Autodesk Inventor part; units mm, degrees
ref_plane "YZ Plane" through (0, 0, 0) normal (1, 0, 0) x (0, 1, 0)
ref_plane "XZ Plane" through (0, 0, 0) normal (0, 1, 0) x (-1, 0, 0)
ref_plane "XY Plane" through (0, 0, 0) normal (0, 0, 1) x (1, 0, 0)
sketch "Sketch1" plane through (0, 0, 0) normal (0, 1, 0) x (-1, 0, 0)
  arc A0 (0, 5) -> (0, -5) centre (0, 0) ccw
  arc A1 (-1.6, 1.2) -> (1.6, 1.2) centre (0, 0) ccw
  line L0 (-1.6, 1.2) -> (1.6, 1.2)
  line L1 (95, 124.2688) -> (95, -104.3981) construction
  circle A2 centre (190, 0) radius 11
  arc A3 (179.0531, -6.0345) -> (179.7419, 7.1429) centre (190, 0) ccw
  line L2 (0, -5) -> (177.3016, -5)
  line L3 (0, 5) -> (175.6386, 5)
  arc A4 (179.0531, -6.0345) -> (177.3016, -5) centre (177.3016, -7) ccw
  arc A5 (175.6386, 5) -> (179.7419, 7.1429) centre (175.6386, 10) ccw
  point P0 (178.5436, -5)
  point P1 (178.5436, 5)
  dimension "d2" = 10
  dimension "d3" = 4
  dimension "d4" = 1.2
  dimension "d5" = 95
  dimension "d8" = 22
  dimension "d9" = 25
  dimension "d20" = 2
  dimension "d21" = 5
extrude "Extrusion2" add sketch "Sketch1" along normal blind 10
sketch "Sketch2" plane through (0, 10, 0) normal (0, 1, 0) x (1, 0, 0)
  circle A0 centre (0, 0) radius 2.35
  dimension "d12" = 4.7
extrude "Extrusion3" add sketch "Sketch2" along normal blind 7
sketch "Sketch3" plane through (0, 10, 0) normal (0, 1, 0) x (1, 0, 0)
  circle A0 centre (-190, 0) radius 11 construction
  line L0 (-179, 0) -> (-201, 0) construction
  circle A1 centre (-190, 0) radius 11
  circle A2 centre (-190, 0) radius 3
  point P0 (0, 0)
  dimension "d15" = 22
  dimension "d16" = 22
  dimension "d17" = 6
extrude "Extrusion4" add sketch "Sketch3" against normal blind 3
equation "\"d16\" = d15"
properties part number "eslabon1" material "Plástico ABS"
Can you work these out from the model? Positions are in its coordinate system, mm. A direction names the side the tool comes from. Round coordinates to 2 decimals unless told otherwise and drop trailing zeros. Loops run counter-clockwise (first coordinate to the right, second up) from the corner with the lowest first, then second, coordinate; pieces in that order, holes last. Notation, with made-up numbers: M 9,-39 L 41,-39 A14 ccw 41,-19 Z; hole C -31,81 d5. An arc over 180 degrees is marked long. Write item = value, one per line. Start each with the question number.
(1) Which directions (+Z, -Z, +X, -X, +Y, -Y) give clear straight access to the entire face, cutting with the end or side of a thin tool? Please do faces 5 (the face through (-87, 5, 5)), 6 (the face through (-0.509, 13.451, -2.294)), 7 (the face through (5, 5, 0)), 8 (the face through (-179, 3, 0)), 9 (the face through (-91, 0, 0)).
(2) Suppose I cut it at A-A on x = -190. Write out the boundary of the cut face in (y, z), plus the area to 3 significant figures.
(3) I'm going to push flat-ended pins straight in: P1, Ø4, axis at x = -67.5, y = 7, coming from the +Z side; P2, Ø8, axis at x = -24.5, y = 5.5, coming from the -Z side; P3, Ø7.5, axis at x = -70.5, z = 1.5, coming from the +Y side. Where does each tip first touch, or does it pass through?
(4) I need wall thicknesses on line 1 along X through (y, z) = (4.75, 0); line 2 along Z through (x, y) = (-190, 3); line 3 along Z through (x, y) = (-140, 6.25). Which ranges of each line are inside material? Lowest first, please.
(5) Suppose I cut it at B-B on z = 9. Write out the boundary of the cut face in (x, y).
(6) If we mould it in two halves opening along Z, with no side actions, what happens to faces 1 (the face through (0, 17, 0)), 2 (the face through (-187.14, 8.52, -0.9)), 3 (the face through (-177.98, 4.93, 5.58)), 4 (the face through (-87, 5, -5))? For each: released by +Z, released by -Z, zero draft, split by the parting line, or undercut.
(7) Suppose I cut it at C-C on x = -151. Write out the boundary of the cut face in (y, z), plus the area to 3 significant figures.
Answer block:
q1.face_5 = +Z, +X, +Y, -Y
q1.face_6 = +Y
q1.face_7 = +X, +Y, -Y
q1.face_8 = -Y
q1.face_9 = +Z, -Z, +X, -X, -Y
q2.outline = M 0,-12.5 L 10,-12.5 L 10,-3 L 7,-3 L 7,-11 L 0,-11 Z; M 0,11 L 7,11 L 7,3 L 10,3 L 10,12.5 L 0,12.5 Z
q2.area = 78.0 mm²
q3.P1 = 5
q3.P2 = -5
q3.P3 = 10
q4.line_1 = -202.5 to -201, -179 to -2, 2 to 5
q4.line_2 = -12.5 to -11, 11 to 12.5
q4.line_3 = -5 to 5
q5.outline = M -198.67,0 L -196.32,0 L -196.32,7 L -183.68,7 L -183.68,0 L -181.33,0 L -181.33,10 L -198.67,10 Z
q6.face_1 = zero draft
q6.face_2 = undercut
q6.face_3 = released by +Z
q6.face_4 = released by -Z
q7.outline = M 0,-5 L 10,-5 L 10,5 L 0,5 Z
q7.area = 100 mm²
